```python
from build123d import *

# Parameters (mm, degrees)
F1_R     = 11
F2_DEPTH = 1.5
F4_R     = 6.000001
F5_DEPTH = 0.5
F7_DEPTH = 3


with BuildPart() as f2:
    # F1 (on Top) → F2 (new body)
    with BuildSketch(Plane.XY):
        with Locations((-26.134714, 14.360657)):
            Circle(F1_R)
    extrude(amount=F2_DEPTH)

    # F4 (on face) → F5 (join)
    with BuildSketch(Plane.XY.offset(1.5)):
        with Locations((-26.134714, 14.360657)):
            Circle(F4_R)
    extrude(amount=F5_DEPTH)

    # F6 (on face) → F7 (join)
    with BuildSketch(Plane.XY.offset(2)):
        with BuildLine():
            Line((-25.887165, 10.981324), (-25.887165, 10.476647))
            ThreePointArc((-25.887165, 10.476647), (-23.551928, 11.648914), (-22.463676, 14.024466))
            Line((-22.463676, 14.024466), (-22.966088, 14.024466))
            ThreePointArc((-22.966088, 14.024466), (-23.905454, 12.002628), (-25.887165, 10.981324))
        make_face()
        with BuildLine():
            ThreePointArc((-26.887165, 10.981324), (-28.868875, 12.002628), (-29.808241, 14.024466))
            Line((-29.808241, 14.024466), (-30.310653, 14.024466))
            ThreePointArc((-30.310653, 14.024466), (-29.222401, 11.648914), (-26.887165, 10.476647))
            Line((-26.887165, 10.476647), (-26.887165, 10.981324))
        make_face()
        with BuildLine():
            ThreePointArc((-29.808241, 14.745119), (-28.868875, 16.766958), (-26.887165, 17.788262))
            Line((-26.887165, 17.788262), (-26.887165, 18.292938))
            ThreePointArc((-26.887165, 18.292938), (-29.222401, 17.120671), (-30.310653, 14.745119))
            Line((-30.310653, 14.745119), (-29.808241, 14.745119))
        make_face()
        with BuildLine():
            Line((-22.966088, 14.745119), (-22.463676, 14.745119))
            ThreePointArc((-22.463676, 14.745119), (-23.551928, 17.120671), (-25.887165, 18.292938))
            Line((-25.887165, 18.292938), (-25.887165, 17.788262))
            ThreePointArc((-25.887165, 17.788262), (-23.905454, 16.766958), (-22.966088, 14.745119))
        make_face()
    extrude(amount=F7_DEPTH)


solid = f2.part
```
CAD build for the part. Positions are in the model's coordinates, mm. A direction names the side the tool comes from. Coordinates: 2 decimals unless noted, no trailing zeros. Order: outer loops, then holes, each group sorted by start corner. A loop starts at its lowest first (then second) coordinate and runs counter-clockwise, first axis right, second up. Notation, with made-up numbers: (-6, 29.25) -> (28, 29.25) arc R20 cw to (28, 61.25) -> close; hole circle Ø5 at (7.5, 66.5). An arc over 180 degrees is marked (long way). Use one line per item in the form item = value. Start each with the question number.
1) Drill centre lines: L1, parallel to Z at x = -28, y = 4.5; L2, parallel to Z at x = -28.25, y = 9.25; L3, parallel to X at y = 16.25, z = 4.05. Where is each one in solid material? Low to high. Write a range as [from, to].
2) Pull direction X, two halves, no side cores. Call faces 1 (the flat face through (-23.7, 12, 5)), 2 (the cylindrical face through (-29.196, 17.147, 3.479)), 3 (the cylindrical face through (-28.847, 11.98, 3.479)), 4 (the cylindrical face through (-27.435, 8.503, 1.746)): +X half, -X half, draft (parallel to the pull), parting line (faces both ways), or undercut.
3) Drop flat-ended pins along their axis: pin 1 (0.6 mm diameter, centred on x = -22.5, z = 4, fed in from +Y); pin 2 (0.6 mm diameter, centred on x = -23, z = 3, fed in from -Y); pin 3 (2 mm diameter, centred on x = -29.5, z = 2, fed in from +Y). Give the stop position or say it passes through.
4) Band-saw the part on A-A on z = 4.3. Give the cut face in (x, y), then the cut area to 3 significant figures.
5) Band-saw the part on B-B on y = 15.75. Give the cut face in (x, z), then the cut area to 3 significant figures.
6) Band-saw the part on D-D on x = -21. Give the cut face in (y, z), then the cut area to 3 significant figures.
7) Tool access for faces 5 (the cylindrical face through (-23.526, 17.094, 3.479)), 6 (the cylindrical face through (-29.25, 11.68, 3.48)), 7 (the cylindrical face through (-23.93, 16.79, 3.48)), 8 (the cylindrical face through (-23.6, 11.6, 3.5)): list every direction of +Z, -Z, +X, -X, +Y, -Y with a clear straight run to the whole face (end or side of a thin tool).
8) Band-saw the part on C-C on x = -28.5. Give the cut face in (y, z).
Entries:
q1.L1 = [0, 1.5]
q1.L2 = [0, 2]
q1.L3 = [-29.86, -29.28], [-23.5, -22.92]
q2.face_1 = draft
q2.face_2 = -X half
q2.face_3 = undercut
q2.face_4 = parting line
q3.pin_1 = 16.01
q3.pin_2 = 11.94
q3.pin_3 = 25.07
q4.outline = (-30.31, 14.02) arc R3.94 ccw to (-26.89, 10.48) -> (-26.89, 10.98) arc R3.44 cw to (-29.81, 14.02) -> close; (-30.31, 14.75) -> (-29.81, 14.75) arc R3.44 cw to (-26.89, 17.79) -> (-26.89, 18.29) arc R3.94 ccw to start; (-25.89, 10.48) arc R3.94 ccw to (-22.46, 14.02) -> (-22.97, 14.02) arc R3.44 cw to (-25.89, 10.98) -> close; (-25.89, 17.79) arc R3.44 cw to (-22.97, 14.75) -> (-22.46, 14.75) arc R3.94 ccw to (-25.89, 18.29) -> close
q4.area = 9.87 mm2
q5.outline = (-37.05, 0) -> (-15.22, 0) -> (-15.22, 1.5) -> (-20.3, 1.5) -> (-20.3, 2) -> (-22.69, 2) -> (-22.69, 5) -> (-23.23, 5) -> (-23.23, 2) -> (-29.54, 2) -> (-29.54, 5) -> (-30.08, 5) -> (-30.08, 2) -> (-31.97, 2) -> (-31.97, 1.5) -> (-37.05, 1.5) -> close
q5.area = 41.8 mm2
q6.outline = (4.63, 0) -> (24.09, 0) -> (24.09, 1.5) -> (17.46, 1.5) -> (17.46, 2) -> (11.26, 2) -> (11.26, 1.5) -> (4.63, 1.5) -> close
q6.area = 32.3 mm2
q7.face_5 = +Z, +X, +Y
q7.face_6 = +Z, -X, -Y
q7.face_7 = +Z
q7.face_8 = +Z, +X, -Y
q8.outline = (3.62, 0) -> (25.1, 0) -> (25.1, 1.5) -> (19.87, 1.5) -> (19.87, 2) -> (17.71, 2) -> (17.71, 5) -> (17.1, 5) -> (17.1, 2) -> (11.67, 2) -> (11.67, 5) -> (11.06, 5) -> (11.06, 2) -> (8.85, 2) -> (8.85, 1.5) -> (3.62, 1.5) -> close
